```python
from build123d import *

# Parameters (mm, degrees)
SKETCH1_W           = 90
SKETCH1_H           = 58
BOSS_EXTRUDE1_DEPTH = 20
SKETCH2_R           = 1.5
CUT_EXTRUDE1_DEPTH  = 20
SKETCH3_W           = 20
SKETCH3_H           = 10
BOSS_EXTRUDE2_DEPTH = 40
SKETCH4_W           = 20
SKETCH4_H           = 20
BOSS_EXTRUDE3_DEPTH = 40


with BuildPart() as part:
    # Sketch1 → Boss-Extrude1 (new body)
    with BuildSketch(Plane(origin=(0, 0, 0), x_dir=(1, 0, 0), z_dir=(0, 1, 0))):
        Rectangle(SKETCH1_W, SKETCH1_H)
    extrude(amount=BOSS_EXTRUDE1_DEPTH)

    # Sketch2 → Cut-Extrude1 (cut)
    with BuildSketch(Plane(origin=(0, 20, 0), x_dir=(1, 0, 0), z_dir=(0, 1, 0))):
        with Locations((42, 24.5)):
            Circle(SKETCH2_R)
        with Locations((42, -24.5)):
            Circle(SKETCH2_R)
        with Locations((-16, 24.5)):
            Circle(SKETCH2_R)
        with Locations((-16, -24.5)):
            Circle(SKETCH2_R)
    extrude(amount=-CUT_EXTRUDE1_DEPTH, mode=Mode.SUBTRACT)

    # Sketch3 → Boss-Extrude2 (add)
    with BuildSketch(Plane(origin=(0, 0, -29), x_dir=(-1, 0, 0), z_dir=(0, 0, -1))):
        with Locations((-35, 5)):
            Rectangle(SKETCH3_W, SKETCH3_H)
    extrude(amount=BOSS_EXTRUDE2_DEPTH)

    # Sketch4 → Boss-Extrude3 (add)
    with BuildSketch(Plane.ZY.offset(45)):
        with Locations((0.272543659, 10)):
            Rectangle(SKETCH4_W, SKETCH4_H)
    extrude(amount=BOSS_EXTRUDE3_DEPTH)


solid = part.part
```
Can you work these out from the model? Positions are in its coordinate system, mm. A direction names the side the tool comes from. Coordinates: 2 decimals unless noted, no trailing zeros. Loops run counter-clockwise (first coordinate to the right, second up) from the corner with the lowest first, then second, coordinate; pieces in that order, holes last. Notation, with made-up numbers: (82, 69) -> (116, 69) arc R27 cw to (116, 107) -> close; hole circle Ø5 at (12.25, 77.5). An arc over 180 degrees is marked (long way). Put each result on its own line as item: value. Start each with the question number.
Q1. If I drill on line 1 (Z direction, x = -16, y = 4.25); line 2 (X direction, y = 8.25, z = 24.5); line 3 (Z direction, x = 42, y = 5.5), over which ranges is the centre line in solid material (lowest first)? Write a range as [from, to].
Q2. Thinking about a two-plate mould opening in X: for faces 1 (the face through (45, 8, -8)), 2 (the face through (-5, 0, -8)), 3 (the face through (-17.11, 10.14, -25.51)), 4 (the face through (-45, 10, -19)), which applies, pulls with the +X half, pulls with the -X half, needs draft (parallel to the pull), parting line crosses it, or undercut?
Q3. I want a section at D-D (x = -16). Write out the boundary of the cut face in (y, z), plus the area to 3 significant figures.
Q4. I want a section at C-C (x = 42). Write out the boundary of the cut face in (y, z), plus the area to 3 significant figures.
Q5. For faces 5 (the face through (35, 10, -49)), 6 (the face through (-6, 20, 0)), 7 (the face through (-45, 10, 20)), 8 (the face through (25, 5, -49)), 9 (the face through (35, 5, -69)), which set-ups out of +Z, -Z, +X, -X, +Y, -Y let a thin tool reach every point of the face, with its end or its side?
Q6. I want a section at A-A (z = 24.5). Write out the boundary of the cut face in (x, y).
Q7. I want a section at B-B (y = 8.5). Write out the boundary of the cut face in (x, z).
Q8. I'm going to push flat-ended pins straight in: P1, Ø6, axis at y = 10, z = -20, coming from the -X side; P2, Ø2.5, axis at x = -16, z = -24.5, coming from the +Y side; P3, Ø11, axis at y = 7, z = -47.5, coming from the -X side; P4, Ø6, axis at x = 31.5, z = -44, coming from the +Y side. Where does each tip first touch, or does it pass through?
Taken from the geometry:
1. line 1: z = [-29, -26], [-23, 23], [26, 29]
1. line 2: x = [-45, -17.5], [-14.5, 40.5], [43.5, 45]
1. line 3: z = [-69, -26], [-23, 23], [26, 29]
2. face 1: pulls with the +X half
2. face 2: needs draft
2. face 3: undercut
2. face 4: pulls with the -X half
3. outline: (0, -29) -> (20, -29) -> (20, -26) -> (0, -26) -> close; (0, -23) -> (20, -23) -> (20, 23) -> (0, 23) -> close; (0, 26) -> (20, 26) -> (20, 29) -> (0, 29) -> close
3. area: 1,040 mm2
4. outline: (0, -69) -> (10, -69) -> (10, -29) -> (20, -29) -> (20, -26) -> (0, -26) -> close; (0, -23) -> (20, -23) -> (20, 23) -> (0, 23) -> close; (0, 26) -> (20, 26) -> (20, 29) -> (0, 29) -> close
4. area: 1,440 mm2
5. face 5: -Z, +X, -X, +Y
5. face 6: +Z, -Z, +X, -X, +Y
5. face 7: +Z, -X, +Y, -Y
5. face 8: -Z, -X, +Y, -Y
5. face 9: -Z, +X, -X, +Y, -Y
6. outline: (-45, 0) -> (-17.5, 0) -> (-17.5, 20) -> (-45, 20) -> close; (-14.5, 0) -> (40.5, 0) -> (40.5, 20) -> (-14.5, 20) -> close; (43.5, 0) -> (45, 0) -> (45, 20) -> (43.5, 20) -> close
7. outline: (-85, -9.73) -> (-45, -9.73) -> (-45, -29) -> (25, -29) -> (25, -69) -> (45, -69) -> (45, 29) -> (-45, 29) -> (-45, 10.27) -> (-85, 10.27) -> close; hole circle Ø3 at (-16, -24.5); hole circle Ø3 at (-16, 24.5); hole circle Ø3 at (42, -24.5); hole circle Ø3 at (42, 24.5)
8. P1: stops at x = -45
8. P2: passes through
8. P3: stops at x = 25
8. P4: stops at y = 10
